CAD build for the part. Positions are in the model's coordinates, mm. Face numbers are marked on the shaded views. A direction names the side the tool comes from. Round coordinates to 2 decimals unless told otherwise and drop trailing zeros. Write each loop counter-clockwise with the first axis right and the second up, starting at its lowest first coordinate (ties: lowest second). Pieces come first, ordered by that corner, then holes. Notation, with made-up numbers: M 77,47 L 104,47 A12 cw 104,60 Z; hole C -8.75,31 d1. An arc over 180 degrees is marked long. Write each question's results on one line, items separated by ' | '. Start each with the question number.
```python
from build123d import *

# Parameters (mm, degrees)
ESQUISSE1_W              = 100
ESQUISSE1_H              = 100
BOSS_EXTRU_1_DEPTH       = 6
ESQUISSE2_W              = 30
ESQUISSE2_H              = 100
BOSS_EXTRU_2_DEPTH       = 6
ESQUISSE3_W              = 30
ESQUISSE3_H              = 100
BOSS_EXTRU_3_DEPTH       = 6
ESQUISSE4_W              = 6
ESQUISSE4_H              = 100
BOSS_EXTRU_4_DEPTH       = 40
ESQUISSE5_W              = 6
ESQUISSE5_H              = 100
BOSS_EXTRU_5_DEPTH       = 40
BOSS_EXTRU_7_DEPTH       = 100
BOSS_EXTRU_8_DEPTH       = 100
ESQUISSE9_R              = 1
ENL_V_MAT_EXTRU_1_DEPTH  = 60
ESQUISSE10_R             = 4
ENL_V_MAT_EXTRU_2_DEPTH  = 17
BOSS_EXTRU_27_DEPTH      = 6
BOSS_EXTRU_27_DEPTH_BACK = 3
ESQUISSE28_W             = 100
ESQUISSE28_H             = 30
ESQUISSE29_W             = 100
ESQUISSE29_H             = 6
BOSS_EXTRU_28_DEPTH      = 40
BOSS_EXTRU_30_DEPTH      = 6
BOSS_EXTRU_30_DEPTH_BACK = 3
ESQUISSE30_W             = 100
ESQUISSE30_H             = 30
ESQUISSE31_W             = 100
ESQUISSE31_H             = 6
BOSS_EXTRU_31_DEPTH      = 40
BOSS_EXTRU_32_DEPTH      = 100
BOSS_EXTRU_33_DEPTH      = 100
ESQUISSE34_R             = 1
ENL_V_MAT_EXTRU_7_DEPTH  = 100
ESQUISSE35_R             = 4
ENL_V_MAT_EXTRU_8_DEPTH  = 17
ESQUISSE36_R             = 25
ENL_V_MAT_EXTRU_9_DEPTH  = 6
ESQUISSE37_W             = 100
ESQUISSE37_H             = 94.110781927
BOSS_EXTRU_34_DEPTH      = 24


with BuildPart() as part:
    # Esquisse1 → Boss.-Extru.1 (new body)
    with BuildSketch(Plane.XY):
        Rectangle(ESQUISSE1_W, ESQUISSE1_H)
    extrude(amount=BOSS_EXTRU_1_DEPTH)

    # Esquisse2 → Boss.-Extru.2 (add)
    with BuildSketch(Plane.ZY.offset(50)):
        with Locations((-9, 0)):
            Rectangle(ESQUISSE2_W, ESQUISSE2_H)
    extrude(amount=BOSS_EXTRU_2_DEPTH)

    # Esquisse3 → Boss.-Extru.3 (add)
    with BuildSketch(Plane(origin=(50, 0, 0), x_dir=(0, 0, -1), z_dir=(1, 0, 0))):
        with Locations((9, 0)):
            Rectangle(ESQUISSE3_W, ESQUISSE3_H)
    extrude(amount=BOSS_EXTRU_3_DEPTH)

    # Esquisse4 → Boss.-Extru.4 (add)
    with BuildSketch(Plane(origin=(56, 0, 0), x_dir=(0, 0, -1), z_dir=(1, 0, 0))):
        with Locations((21, 0)):
            Rectangle(ESQUISSE4_W, ESQUISSE4_H)
    extrude(amount=BOSS_EXTRU_4_DEPTH)

    # Esquisse5 → Boss.-Extru.5 (add)
    with BuildSketch(Plane.ZY.offset(56)):
        with Locations((-21, 0)):
            Rectangle(ESQUISSE5_W, ESQUISSE5_H)
    extrude(amount=BOSS_EXTRU_5_DEPTH)

    # Esquisse6 → Boss.-Extru.7 (add)
    with BuildSketch(Plane(origin=(0, 50, 0), x_dir=(1, 0, 0), z_dir=(0, 1, 0))):
        Polygon((-56, -6), (-56, 18), (-96, 18), align=None)
    extrude(amount=-BOSS_EXTRU_7_DEPTH)

    # Esquisse8 → Boss.-Extru.8 (add)
    with BuildSketch(Plane(origin=(0, -50, 0), x_dir=(-1, 0, 0), z_dir=(0, -1, 0))):
        Polygon((-56, -6), (-96, 18), (-56, 18), align=None)
    extrude(amount=-BOSS_EXTRU_8_DEPTH)

    # Esquisse9 → Enlèv. mat.-Extru.1 (cut)
    with BuildSketch(Plane(origin=(0, 0, -24), x_dir=(-1, 0, 0), z_dir=(0, 0, -1))):
        with Locations((-76, 30)):
            Circle(ESQUISSE9_R)
        with Locations((-76, -30)):
            Circle(ESQUISSE9_R)
        with Locations((76, -30)):
            Circle(ESQUISSE9_R)
        with Locations((76, 30)):
            Circle(ESQUISSE9_R)
    extrude(amount=-ENL_V_MAT_EXTRU_1_DEPTH, mode=Mode.SUBTRACT)

    # Esquisse10 → Enlèv. mat.-Extru.2 (cut)
    with BuildSketch(Plane.XY.offset(6)):
        with Locations((76, 30)):
            Circle(ESQUISSE10_R)
        with Locations((76, -30)):
            Circle(ESQUISSE10_R)
        with Locations((-76, -30)):
            Circle(ESQUISSE10_R)
        with Locations((-76, 30)):
            Circle(ESQUISSE10_R)
    extrude(amount=-ENL_V_MAT_EXTRU_2_DEPTH, mode=Mode.SUBTRACT)

    # Esquisse28 → Boss.-Extru.27 (add, two sides: drawn at the far end of the back side and taken through both)
    with BuildSketch(Plane(origin=(0, -50, 0), x_dir=(-1, 0, 0), z_dir=(0, -1, 0)).offset(-BOSS_EXTRU_27_DEPTH_BACK)):
        with Locations((0, 9)):
            Rectangle(ESQUISSE28_W, ESQUISSE28_H)
    extrude(amount=BOSS_EXTRU_27_DEPTH + BOSS_EXTRU_27_DEPTH_BACK)

    # Esquisse29 → Boss.-Extru.28 (add)
    with BuildSketch(Plane(origin=(0, -56, 0), x_dir=(-1, 0, 0), z_dir=(0, -1, 0))):
        with Locations((0, 21)):
            Rectangle(ESQUISSE29_W, ESQUISSE29_H)
    extrude(amount=BOSS_EXTRU_28_DEPTH)

    # Esquisse30 → Boss.-Extru.30 (add, two sides: drawn at the far end of the back side and taken through both)
    with BuildSketch(Plane(origin=(0, 50, 0), x_dir=(1, 0, 0), z_dir=(0, 1, 0)).offset(-BOSS_EXTRU_30_DEPTH_BACK)):
        with Locations((0, 9)):
            Rectangle(ESQUISSE30_W, ESQUISSE30_H)
    extrude(amount=BOSS_EXTRU_30_DEPTH + BOSS_EXTRU_30_DEPTH_BACK)

    # Esquisse31 → Boss.-Extru.31 (add)
    with BuildSketch(Plane(origin=(0, 56, 0), x_dir=(1, 0, 0), z_dir=(0, 1, 0))):
        with Locations((0, 21)):
            Rectangle(ESQUISSE31_W, ESQUISSE31_H)
    extrude(amount=BOSS_EXTRU_31_DEPTH)

    # Esquisse32 → Boss.-Extru.32 (add)
    with BuildSketch(Plane.ZY.offset(50)):
        Polygon((-18, -56), (6, -56), (-18, -96), align=None)
    extrude(amount=-BOSS_EXTRU_32_DEPTH)

    # Esquisse33 → Boss.-Extru.33 (add)
    with BuildSketch(Plane.ZY.offset(50)):
        Polygon((-18, 56), (6, 56), (-18, 96), align=None)
    extrude(amount=-BOSS_EXTRU_33_DEPTH)

    # Esquisse34 → Enlèv. mat.-Extru.7 (cut)
    with BuildSketch(Plane.XY.offset(6)):
        with Locations(Location((-35.892206296, -76, 0), (0, 0, 90))):
            Circle(ESQUISSE34_R)
        with Locations(Location((33.387808828, -76, 0), (0, 0, 90))):
            Circle(ESQUISSE34_R)
        with Locations(Location((33.387808828, 76, 0), (0, 0, 270))):
            Circle(ESQUISSE34_R)
        with Locations(Location((-35.892206296, 76, 0), (0, 0, 270))):
            Circle(ESQUISSE34_R)
    extrude(amount=-ENL_V_MAT_EXTRU_7_DEPTH, mode=Mode.SUBTRACT)

    # Esquisse35 → Enlèv. mat.-Extru.8 (cut)
    with BuildSketch(Plane.XY.offset(6)):
        with Locations((33.387808828, -76)):
            Circle(ESQUISSE35_R)
        with Locations((-35.892206296, -76)):
            Circle(ESQUISSE35_R)
        with Locations(Location((-35.892206296, 76, 0), (0, 0, 270))):
            Circle(ESQUISSE35_R)
        with Locations(Location((33.387808828, 76, 0), (0, 0, 270))):
            Circle(ESQUISSE35_R)
    extrude(amount=-ENL_V_MAT_EXTRU_8_DEPTH, mode=Mode.SUBTRACT)

    # Esquisse36 → Enlèv. mat.-Extru.9 (cut)
    with BuildSketch(Plane.XY.offset(6)):
        Circle(ESQUISSE36_R)
    extrude(amount=-ENL_V_MAT_EXTRU_9_DEPTH, mode=Mode.SUBTRACT)

    # Esquisse37 → Boss.-Extru.34 (add)
    with BuildSketch(Plane(origin=(0, 0, -24), x_dir=(-1, 0, 0), z_dir=(0, 0, -1))):
        with Locations((0, 0.055390964)):
            Rectangle(ESQUISSE37_W, ESQUISSE37_H)
    extrude(amount=-BOSS_EXTRU_34_DEPTH)


solid = part.part
```
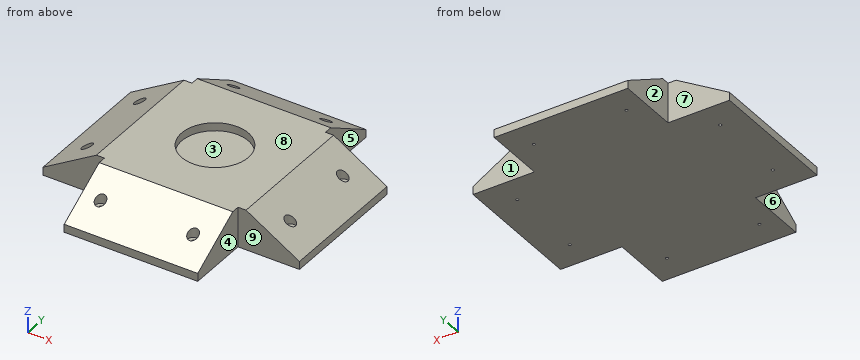
1) Wall check: line 1 along X through (y, z) = (-76, -13.75); line 2 along X through (y, z) = (76, -8); line 3 along Y through (x, z) = (-76, -7.25). Give the ranges that are in metal, low to high. Write a range as from..to.
2) Saw through at C-C, the plane z = 2.5. Write the cut outline in (x, y), plus the area to 3 significant figures.
3) 3-axis set-ups, long thin cutter, end or side, ignore diameter. For the marked faces 5, 6, 7, 8 and 9: which of +Z, -Z, +X, -X, +Y, -Y reach the whole face in a straight line?
4) Drop flat-ended pins along their axis: pin 1 Ø2.5 at (x, y) = (-36.5, -74.5) entering from +Z; pin 2 Ø9 at (x, y) = (75, 28) entering from +Z; pin 3 Ø1.5 at (x, y) = (-61.5, 38.5) entering from +Z; pin 4 Ø10.5 at (x, y) = (33.39, 76) entering from -Z. Give the stop position or say it passes through.
5) Pull direction X, two halves, no side cores. Call the marked faces 1, 2, 3 and 4: pulls with the +X half, pulls with the -X half, needs draft (parallel to the pull), parting line crosses it, or undercut.
6) Saw through at B-B, the plane z = -20.5. State how many separate pieces and enclosed holes the cut face has, plus the area to 3 significant figures.
7) Saw through at A-A, the plane x = 0. Write the cut outline in (y, z), plus the area to 3 significant figures.
Filled sheet:
1) line 1: x = -50..-36.89, -34.89..32.39, 34.39..50 | line 2: x = -50..-39.89, -31.89..29.39, 37.39..50 | line 3: y = -50..-34, -26..26, 34..50
2) outline: M -61.83,-50 L -50,-50 L -50,-61.83 L 50,-61.83 L 50,-50 L 61.83,-50 L 61.83,50 L 50,50 L 50,61.83 L -50,61.83 L -50,50 L -61.83,50 Z; hole C 0,0 d50 | area: 12,800 mm^2
3) face 5: +Z, -Z, +X, +Y | face 6: +Z, -Z, -X, -Y | face 7: +Z, -Z, -X, +Y | face 8: +Z, +X, -X, +Y, -Y | face 9: +Z, -Z, +X, -Y
4) pin 1: stops at z = -11 | pin 2: stops at z = -2.7 | pin 3: stops at z = 3.15 | pin 4: stops at z = -24
5) face 1: needs draft | face 2: pulls with the -X half | face 3: undercut | face 4: pulls with the +X half
6) separate pieces: 1 | enclosed holes: 8 | area: 28,400 mm^2
7) outline: M -96,-24 L 96,-24 L 96,-18 L 56,6 L 25,6 L 25,0 L -25,0 L -25,6 L -56,6 L -96,-18 Z | area: 4,500 mm^2
